Source: CAD feature listing. Evaluate the final solid. Frame: model axes, mm. Face numbers are marked on the shaded views. A direction names the side the tool comes from. Round coordinates to 2 decimals unless told otherwise and drop trailing zeros. Order: outer loops, then holes, each group sorted by start corner. A loop starts at its lowest first (then second) coordinate and runs counter-clockwise, first axis right, second up. Notation, with made-up numbers: (49.5, 33.5) - (96.5, 33.5) arc R24 cw to (96.5, 68.5) - close; hole circle Ø6 at (-11.75, -8.75). An arc over 180 degrees is marked (long way). Return JSON: item names as keys, results as strings. Group by question number.
1) Ray query, line 1 (Y direction, x = 6.75, z = 5.75); line 2 (X direction, y = -5, z = 12.5); line 3 (Y direction, x = 4.25, z = 20.5). Return the intervals inside material, ascending. Write a range as from..to.
2) Section C-C, the plane x = 7.25. Return loops of the section in (y, z).
3) Section A-A, the plane z = 11.75. Return loops of the section in (x, y).
4) Mould query, pull axis Y, two halves, no side actions, for the marked faces 1, 2 and 3. Classes: pulls with the +Y half, pulls with the -Y half, needs draft (parallel to the pull), parting line crosses it, or undercut.
5) Access query for the marked faces 4, 5, 6 and 7. Directions: +Z, -Z, +X, -X, +Y, -Y. A direction counts if a zero-diameter tool reaches every point of the face in a straight line with its end or side. Return the directions, or none.
6) Contact query for flat-ended pins moving along their axis: P1, Ø2, axis at x = 3, z = 16.5, coming from the -Y side; P2, Ø4, axis at x = 1.5, y = 6, coming from the +Z side; P3, Ø6, axis at x = -4, z = 14.5, coming from the +Y side. Output: stop coordinate, or through.
7) Section B-B, the plane y = 11. Return loops of the section in (x, z), plus the area to 3 significant figures.
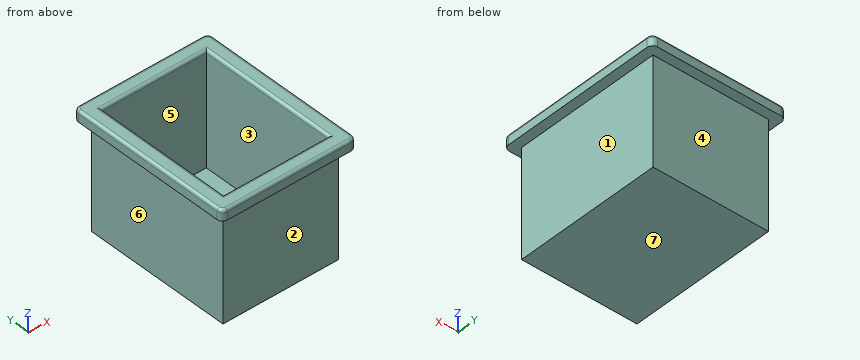
```python
from build123d import *

# Parameters (mm, degrees)
SKETCH1_W           = 21.5
SKETCH1_H           = 27.5
BOSS_EXTRUDE1_DEPTH = 20
SKETCH2_W           = 25
SKETCH2_H           = 31
BOSS_EXTRUDE2_DEPTH = 2
SKETCH3_W           = 19.5
SKETCH3_H           = 25.5
CUT_EXTRUDE1_DEPTH  = 21
FILLET1_R           = 1
FILLET2_R           = 0.5


with BuildPart() as part:
    # Sketch1 → Boss-Extrude1 (new body)
    with BuildSketch(Plane.XY):
        Rectangle(SKETCH1_W, SKETCH1_H)
    extrude(amount=BOSS_EXTRUDE1_DEPTH)

    # Sketch2 → Boss-Extrude2 (add)
    with BuildSketch(Plane.XY.offset(20)):
        Rectangle(SKETCH2_W, SKETCH2_H)
    extrude(amount=BOSS_EXTRUDE2_DEPTH)

    # Sketch3 → Cut-Extrude1 (cut)
    with BuildSketch(Plane.XY.offset(22)):
        Rectangle(SKETCH3_W, SKETCH3_H)
    extrude(amount=-CUT_EXTRUDE1_DEPTH, mode=Mode.SUBTRACT)

    # Fillet1
    fillet1_edges = [part.edges().sort_by_distance(p)[0] for p in [
        (12.5, -15.5, 21),
        (12.5, 15.5, 21),
        (-12.5, 15.5, 21),
        (-12.5, -15.5, 21),
    ]]
    fillet(fillet1_edges, radius=FILLET1_R)

    # Fillet2
    fillet2_edges = [part.edges().sort_by_distance(p)[0] for p in [
        (9.75, 0, 22),
        (0, 12.75, 22),
        (-9.75, 0, 22),
        (0, -12.75, 22),
        (0, -15.5, 22),
        (-12.5, 0, 22),
        (12.5, 0, 22),
        (0, 15.5, 22),
        (12.207106781, 15.207106781, 22),
        (-12.207106781, 15.207106781, 22),
        (12.207106781, -15.207106781, 22),
        (-12.207106781, -15.207106781, 22),
    ]]
    fillet(fillet2_edges, radius=FILLET2_R)


solid = part.part
```
Geometry check:
{
 "1": {"line 1": "-13.75..-12.75, 12.75..13.75", "line 2": "-10.75..-9.75, 9.75..10.75", "line 3": "-15.5..-12.75, 12.75..15.5"},
 "2": {"outline": "(-15.5, 20) - (-13.75, 20) - (-13.75, 0) - (13.75, 0) - (13.75, 20) - (15.5, 20) - (15.5, 21.5) arc R0.5 ccw to (15, 22) - (13.25, 22) arc R0.5 ccw to (12.75, 21.5) - (12.75, 1) - (-12.75, 1) - (-12.75, 21.5) arc R0.5 ccw to (-13.25, 22) - (-15, 22) arc R0.5 ccw to (-15.5, 21.5) - close"},
 "3": {"outline": "(-10.75, -13.75) - (10.75, -13.75) - (10.75, 13.75) - (-10.75, 13.75) - close; hole (-9.75, -12.75) - (9.75, -12.75) - (9.75, 12.75) - (-9.75, 12.75) - close"},
 "4": {"face 1": "needs draft", "face 2": "pulls with the -Y half", "face 3": "undercut"},
 "5": {"face 4": "-Z, +X, -X, +Y", "face 5": "+Z", "face 6": "-Z, -X, +Y, -Y", "face 7": "-Z, +X, -X, +Y, -Y"},
 "6": {"P1": "y = -13.75", "P2": "z = 1", "P3": "y = 13.75"},
 "7": {"outline": "(-12.5, 20) - (-10.75, 20) - (-10.75, 0) - (10.75, 0) - (10.75, 20) - (12.5, 20) - (12.5, 21.5) arc R0.5 ccw to (12, 22) - (10.25, 22) arc R0.5 ccw to (9.75, 21.5) - (9.75, 1) - (-9.75, 1) - (-9.75, 21.5) arc R0.5 ccw to (-10.25, 22) - (-12, 22) arc R0.5 ccw to (-12.5, 21.5) - close", "area": "70.3 mm2"}
}
